Model file for the job. Use its own axes, mm. A direction names the side the tool comes from. Coordinates: 2 decimals unless noted, no trailing zeros. Order: outer loops, then holes, each group sorted by start corner. A loop starts at its lowest first (then second) coordinate and runs counter-clockwise, first axis right, second up. Notation, with made-up numbers: (-21.75, 57) -> (10.25, 57) arc R9 ccw to (10.25, 62) -> close; hole circle Ø10 at (-1.5, -15.75). An arc over 180 degrees is marked (long way). Return JSON: item names as keys, results as strings. Group by question number.
1) Cut at A-A (x = 19). Write the cut outline in (y, z), and give its area (3 significant figures).
2) Which spindle directions (+Z, -Z, +X, -X, +Y, -Y) get a long thin tool onto all of the face, cutting with end or side? Do faces 4 (the cylindrical face through (4.1, 1, 0)), 5 (the flat face through (7, 1, -10)). Say none if no direction does.
3) Flat gauge pin, fed straight in: pin 1 (1.4 mm diameter, centred on x = 19, z = 4.75, fed in from +Y). Where does the tip first touch, or does it go through?
4) Pull direction X, two halves, no side cores. Call faces 1 (the flat face through (7, 1, 10)), 2 (the cylindrical face through (18.152, 0.986, 3.973)), 3 (the cylindrical face through (23.1, 1.01, -9.14)): +X half, -X half, draft (parallel to the pull), parting line (faces both ways), or undercut.
5) Probe line 1 (Z direction, x = 19, y = 0.45); line 2 (X direction, y = 1.65, z = -4.75); line 3 (Z direction, x = 2, y = 0.85). List the from-to ranges inside material, lowest first.
6) Cut at C-C (y = 0.6). Write the cut outline in (x, z), and give its area (3 significant figures).
7) Cut at D-D (z = 0). Write the cut outline in (x, y).
8) Cut at B-B (z = 4.75). Write the cut outline in (x, y).
from build123d import *

# Parameters (mm, degrees)
SKETCH_1_R          = 1.6
SKETCH_1_R_2        = 1.15
EXTRUDE_1_DEPTH     = 2
FILLET_2_R          = 3
CUT_EXTRUDE_1_DEPTH = 10


with BuildPart() as part:
    # 草图1 → 凸台-拉伸1 (new body)
    with BuildSketch(Plane(origin=(0, 0, 0), x_dir=(1, 0, 0), z_dir=(0, 1, 0))):
        Polygon((-10, 10), (10, 10), (24, 10), (24, -10), (10, -10), (-10, -10), align=None)
        Circle(SKETCH_1_R, mode=Mode.SUBTRACT)
        with Locations((19, -4.75)):
            Circle(SKETCH_1_R_2, mode=Mode.SUBTRACT)
        with Locations((19, 4.75)):
            Circle(SKETCH_1_R_2, mode=Mode.SUBTRACT)
    extrude(amount=EXTRUDE_1_DEPTH)

    # 圆角2
    fillet_2_edges = [part.edges().sort_by_distance(p)[0] for p in [
        (-10, 1, -10),
        (24, 1, -10),
        (24, 1, 10),
        (-10, 1, 10),
    ]]
    fillet(fillet_2_edges, radius=FILLET_2_R)

    # 草图2 → 切除-拉伸1 (cut)
    with BuildSketch(Plane(origin=(0, 2, 0), x_dir=(1, 0, 0), z_dir=(0, 1, 0))):
        with BuildLine():
            Line((2.5, -1.6), (-2.5, -1.6))
            ThreePointArc((-2.5, -1.6), (-4.1, 0), (-2.5, 1.6))
            Line((-2.5, 1.6), (2.5, 1.6))
            ThreePointArc((2.5, 1.6), (4.1, 0), (2.5, -1.6))
        make_face()
    extrude(amount=-CUT_EXTRUDE_1_DEPTH, mode=Mode.SUBTRACT)


solid = part.part
Answers below:
{
 "1": {"outline": "(0, -10) -> (2, -10) -> (2, -5.9) -> (0, -5.9) -> close; (0, -3.6) -> (2, -3.6) -> (2, 3.6) -> (0, 3.6) -> close; (0, 5.9) -> (2, 5.9) -> (2, 10) -> (0, 10) -> close", "area": "30.8 mm^2"},
 "2": {"face 4": "+Y, -Y", "face 5": "-Z, +X, -X, +Y, -Y"},
 "3": {"pin 1": "passes through"},
 "4": {"face 1": "draft", "face 2": "undercut", "face 3": "+X half"},
 "5": {"line 1": "z = -10 to -5.9, -3.6 to 3.6, 5.9 to 10", "line 2": "x = -10 to 17.85, 20.15 to 24", "line 3": "z = -10 to -1.6, 1.6 to 10"},
 "6": {"outline": "(-10, -7) arc R3 ccw to (-7, -10) -> (21, -10) arc R3 ccw to (24, -7) -> (24, 7) arc R3 ccw to (21, 10) -> (-7, 10) arc R3 ccw to (-10, 7) -> close; hole (-2.5, -1.6) -> (2.5, -1.6) arc R1.6 ccw to (2.5, 1.6) -> (-2.5, 1.6) arc R1.6 ccw to start; hole circle Ø2.3 at (19, -4.75); hole circle Ø2.3 at (19, 4.75)", "area": "640 mm^2"},
 "7": {"outline": "(-10, 0) -> (-4.1, 0) -> (-4.1, 2) -> (-10, 2) -> close; (4.1, 0) -> (24, 0) -> (24, 2) -> (4.1, 2) -> close"},
 "8": {"outline": "(-10, 0) -> (17.85, 0) -> (17.85, 2) -> (-10, 2) -> close; (20.15, 0) -> (24, 0) -> (24, 2) -> (20.15, 2) -> close"}
}
